For this review, take the finished solid that the model builds, in its own axes (mm). Face numbers are marked on the shaded views. Give positions to 0.01 mm unless a question says otherwise; leave off trailing zeros. Write each loop counter-clockwise with the first axis right and the second up, starting at its lowest first coordinate (ties: lowest second). Pieces come first, ordered by that corner, then holes.
Q1. For line 1 (X direction, y = 195, z = 13.5); line 2 (Y direction, x = -125, z = 10.25); line 3 (X direction, y = 174.5, z = 5.75), list the stretches that pass through material, from the lowest coordinate up.
Q2. We need section C-C (y = 99.5). Write out the cut boundary in (x, z).
Q3. We need section A-A (z = 6.25). Write out the cut boundary in (x, y), then the cut area to 3 significant figures.
Q4. Mouldability with a two-part tool opening along Y and no side actions: class the marked faces 1, 2 and 3 as released by +Y, released by -Y, zero draft, split by the parting line, or undercut.
Q5. We need section B-B (x = -46). Write out the cut boundary in (y, z), then the cut area to 3 significant figures.
Q6. Insertion check: P1, Ø1.5, axis at x = -107.5, z = 6, coming from the +Y side; P2, Ø2.5, axis at x = -125, y = 195.5, coming from the +Z side; P3, Ø2.5, axis at x = 5, y = 195, coming from the +Z side; P4, Ø3.5, axis at x = -50.5, z = 10, coming from the -Y side. Each pin has a flat end and moves straight along its axis. Give the tip position at first contact, or say it passes through.
```python
from build123d import *

# Parameters (mm, degrees)
BOSS_EXTRUDE1_DEPTH = 4
SKETCH2_W           = 120
SKETCH2_H           = 180
BOSS_EXTRUDE2_DEPTH = 12
SKETCH3_R           = 1.6
CUT_EXTRUDE1_DEPTH  = 12


with BuildPart() as part:
    # Sketch1 → Boss-Extrude1 (new body)
    with BuildSketch(Plane(origin=(0, 0, 0), x_dir=(0, 1, 0), z_dir=(0, 0, 1))):
        with BuildLine():
            Line((-10, 2.4), (-10, 117.6))
            ThreePointArc((-10, 117.6), (-10.702943725, 119.297056275), (-12.4, 120))
            Line((-12.4, 120), (-20, 120))
            Line((-20, 120), (-20, 130))
            Line((-20, 130), (-10, 130))
            Line((-10, 130), (190, 130))
            Line((190, 130), (200, 130))
            Line((200, 130), (200, 120))
            Line((200, 120), (192.4, 120))
            ThreePointArc((192.4, 120), (190.702943725, 119.297056275), (190, 117.6))
            Line((190, 117.6), (190, 2.4))
            ThreePointArc((190, 2.4), (190.702943725, 0.702943725), (192.4, 0))
            Line((192.4, 0), (200, 0))
            Line((200, 0), (200, -10))
            Line((200, -10), (190, -10))
            Line((190, -10), (-10, -10))
            Line((-10, -10), (-20, -10))
            Line((-20, -10), (-20, 0))
            Line((-20, 0), (-12.4, 0))
            ThreePointArc((-12.4, 0), (-10.702943725, 0.702943725), (-10, 2.4))
        make_face()
    extrude(amount=BOSS_EXTRUDE1_DEPTH)

    # Sketch2 → Boss-Extrude2 (add)
    with BuildSketch(Plane.XY.offset(4)):
        with BuildLine():
            Line((10, -20), (10, 200))
            Line((10, 200), (0, 200))
            Line((0, 200), (0, 192.4))
            ThreePointArc((0, 192.4), (-0.702943725, 190.702943725), (-2.4, 190))
            Line((-2.4, 190), (-117.6, 190))
            ThreePointArc((-117.6, 190), (-119.297056275, 190.702943725), (-120, 192.4))
            Line((-120, 192.4), (-120, 200))
            Line((-120, 200), (-130, 200))
            Line((-130, 200), (-130, -20))
            Line((-130, -20), (-120, -20))
            Line((-120, -20), (-120, -12.4))
            ThreePointArc((-120, -12.4), (-119.297056275, -10.702943725), (-117.6, -10))
            Line((-117.6, -10), (-2.4, -10))
            ThreePointArc((-2.4, -10), (-0.702943725, -10.702943725), (0, -12.4))
            Line((0, -12.4), (0, -20))
            Line((0, -20), (10, -20))
        make_face()
        with Locations((-60, 90)):
            Rectangle(SKETCH2_W, SKETCH2_H, mode=Mode.SUBTRACT)
    extrude(amount=BOSS_EXTRUDE2_DEPTH)

    # Sketch3 → Cut-Extrude1 (cut)
    with BuildSketch(Plane.XY.offset(16)):
        with Locations((-125, 195)):
            Circle(SKETCH3_R)
        with Locations((5, 195)):
            Circle(SKETCH3_R)
        with Locations((5, -15)):
            Circle(SKETCH3_R)
        with Locations((-125, -15)):
            Circle(SKETCH3_R)
    extrude(amount=-CUT_EXTRUDE1_DEPTH, mode=Mode.SUBTRACT)


solid = part.part
```
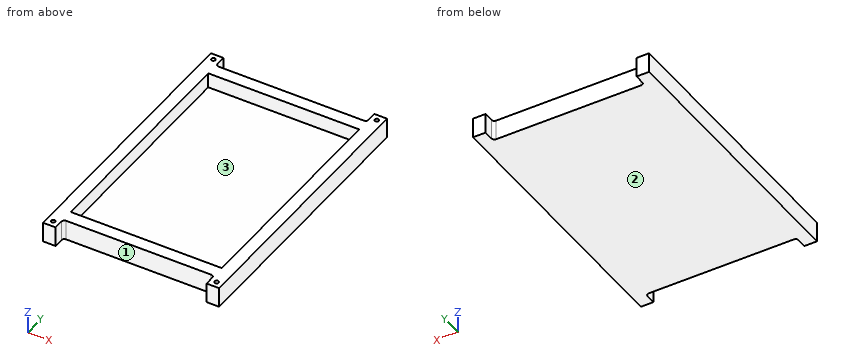
Computed:
1. line 1: x = -130 to -126.6, -123.4 to -120, 0 to 3.4, 6.6 to 10
1. line 2: y = -20 to -16.6, -13.4 to 193.4, 196.6 to 200
1. line 3: x = -130 to -120, 0 to 10
2. outline: (-130, 0) - (10, 0) - (10, 16) - (0, 16) - (0, 4) - (-120, 4) - (-120, 16) - (-130, 16) - close
3. outline: (-130, -20) - (-120, -20) - (-120, -12.4) arc R2.4 cw to (-117.6, -10) - (-2.4, -10) arc R2.4 cw to (0, -12.4) - (0, -20) - (10, -20) - (10, 200) - (0, 200) - (0, 192.4) arc R2.4 cw to (-2.4, 190) - (-117.6, 190) arc R2.4 cw to (-120, 192.4) - (-120, 200) - (-130, 200) - close; hole circle Ø3.2 at (-125, -15); hole circle Ø3.2 at (-125, 195); hole (-120, 0) - (0, 0) - (0, 180) - (-120, 180) - close; hole circle Ø3.2 at (5, -15); hole circle Ø3.2 at (5, 195)
3. area: 6,770 mm2
4. face 1: released by -Y
4. face 2: zero draft
4. face 3: undercut
5. outline: (-10, 0) - (190, 0) - (190, 16) - (180, 16) - (180, 4) - (0, 4) - (0, 16) - (-10, 16) - close
5. area: 1,040 mm2
6. P1: stops at y = 190
6. P2: stops at z = 16
6. P3: stops at z = 4
6. P4: stops at y = -10
